Part model, mm, in its own coordinate system. Face numbers are marked on the shaded views. A direction names the side the tool comes from. Coordinates: 2 decimals unless noted, no trailing zeros. Loops run counter-clockwise (first coordinate to the right, second up) from the corner with the lowest first, then second, coordinate; pieces in that order, holes last. Notation, with made-up numbers: M 55.25,78.5 L 80.25,78.5 A16 cw 80.25,94.5 Z; hole C -24.5,-27.75 d3. An arc over 180 degrees is marked long. Use a Markdown table: item, result. Add a question column.
1) Pull direction X, two halves, no side cores. Call the marked faces 1, 2, 3 and 4: released by +X, released by -X, zero draft, split by the parting line, or undercut.
2) Tool access for the marked faces 5 and 6: list every direction of +Z, -Z, +X, -X, +Y, -Y with a clear straight run to the whole face (end or side of a thin tool).
3) Wall check: probe 1 along Z at (x, y) = (0, -54.75); probe 2 along X at (y, z) = (-6.5, -0.5); probe 3 along Z at (x, y) = (35.5, -24.5). Give the ranges that are in metal, low to high. Write a range as from..to.
4) Pin check, flat tips, straight feed: pin 1 Ø5 at (x, y) = (51.5, -20) entering from +Z; pin 2 Ø1 at (x, y) = (-0.5, -50) entering from -Z; pin 3 Ø10 at (x, y) = (35.5, -37) entering from -Z; pin 4 Ø5 at (x, z) = (0, 0) entering from -Y. Stop position of each tip, or through.
5) Band-saw the part on A-A (y = -7.5). List the corners of the cut face in (x, z).
6) Band-saw the part on B-B (x = -6). List the corners of the cut face in (y, z), plus the area to 3 significant figures.
7) Band-saw the part on D-D (z = 10.5). List the corners of the cut face in (x, y), plus the area to 3 significant figures.
8) Band-saw the part on C-C (y = -34). List the corners of the cut face in (x, z).
from build123d import *

# Parameters (mm, degrees)
F0_R           = 4
F1_DEPTH       = 58
F2_R           = 3.25
F3_DEPTH       = 13.5
F4_R           = 3.25
F5_DEPTH       = 13.5
F8_DEPTH       = 7
F8_DEPTH_BACK  = 7
F9_R           = 6.99999
F11_W          = 19
F11_H          = 3
F12_DEPTH      = 14
F17_R          = 2
F18_DEPTH      = 5
F18_DEPTH_BACK = 0.471687069
F19_R          = 2


# Not quite as in the source:
# - a fillet or chamfer is up to 0.001 mm smaller than in the source, because OpenCascade refuses the exact size


with BuildPart() as f1:
    # F0 (on Front) → F1 (new body)
    with BuildSketch(Plane.XZ):
        Circle(F0_R)
    extrude(amount=F1_DEPTH)

    # F2 (on face) → F3 (cut)
    with BuildSketch(Plane.XZ.offset(58)):
        Circle(F2_R)
    extrude(amount=-F3_DEPTH, mode=Mode.SUBTRACT)

    # F4 (on face) → F5 (cut)
    with BuildSketch(Plane(origin=(0, 0, 0), x_dir=(-1, 0, 0), z_dir=(0, 1, 0))):
        Circle(F4_R)
    extrude(amount=-F5_DEPTH, mode=Mode.SUBTRACT)

    # F7 (on offset) → F8 (join, two sides)
    with BuildSketch(Plane.XZ.offset(29)) as f8_sk:
        with BuildLine():
            Line((0, -1), (0, -4))
            Line((0, -4), (20, -4))
            ThreePointArc((20, -4), (33.4977869164, -1.9540489613), (45.7829596161, 4))
            Line((45.7829596161, 4), (89.0842298053, 29))
            Line((89.0842298053, 29), (87.5842298053, 31.5980762114))
            Line((87.5842298053, 31.5980762114), (44.1796846254, 6.5384503677))
            ThreePointArc((44.1796846254, 6.5384503677), (32.6637808585, 0.9283092986), (20, -1))
            Line((20, -1), (0, -1))
        make_face()
    extrude(amount=F8_DEPTH)
    extrude(f8_sk.sketch, amount=-F8_DEPTH_BACK)

    # F9 (radius 7 in the source; OpenCascade refuses exactly that, so slightly less here)
    f9_edges = [f1.edges().sort_by_distance(p)[0] for p in [
        (88.33423, -36, 30.299038),
        (88.33423, -22, 30.299038),
    ]]
    fillet(f9_edges, radius=F9_R)

    # F11 (on offset) → F12 (join)
    with BuildSketch(Plane(origin=(0, -5, 0), x_dir=(-1, 0, 0), z_dir=(0, 1, 0))):
        with Locations((9.5, 2.5)):
            Rectangle(F11_W, F11_H)
    extrude(amount=-F12_DEPTH)

    # F17 (on 3pt) → F18 (join, two sides)
    with BuildSketch(Plane(origin=(0.602031742, 0, -3.953721561), x_dir=(0.9886047584, 0, 0.1505344865), z_dir=(-0.1505344865, 0, 0.9886047584))) as f18_sk:
        with Locations((29.0842950344, -29.3515790254)):
            Circle(F17_R)
    extrude(amount=F18_DEPTH)
    extrude(f18_sk.sketch, amount=-F18_DEPTH_BACK)

    # F19
    f19_edges = [f1.edges().sort_by_distance(p)[0] for p in [
        (26.625022, -29.351579, 5.066423),
    ]]
    fillet(f19_edges, radius=F19_R)


solid = f1.part
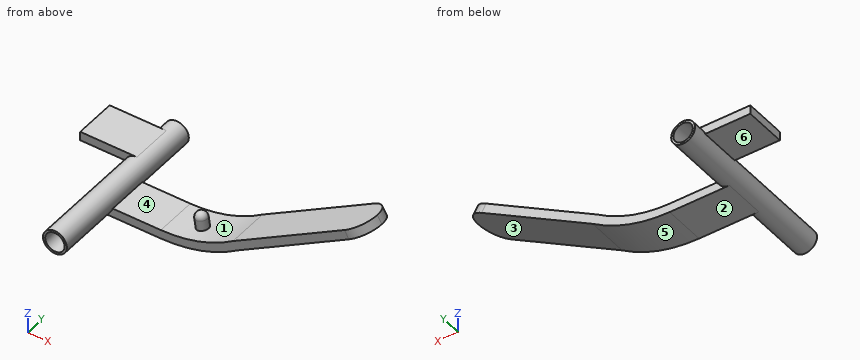
Entries:
| question | item | result |
|---|---|---|
| 1 | face 1 | undercut |
| 1 | face 2 | zero draft |
| 1 | face 3 | released by +X |
| 1 | face 4 | undercut |
| 2 | face 5 | -Z, +X, +Y, -Y |
| 2 | face 6 | -Z, -X, +Y, -Y |
| 3 | probe 1 | -4..-3.25, 3.25..4 |
| 3 | probe 2 | -3.97..-3.21, 3.21..3.97 |
| 3 | probe 3 | -1.28..1.92 |
| 4 | pin 1 | z = 11.63 |
| 4 | pin 2 | z = -4 |
| 4 | pin 3 | z = -2.75 |
| 4 | pin 4 | y = -44.5 |
| 5 | outline | M -19,1 L -3.87,1 A4 ccw long 0,4 L -19,4 Z; hole M -3.09,1 A3.25 ccw long 0,3.25 L 0,1 Z |
| 6 | outline | M -19,1 L -5,1 L -5,4 L -19,4 Z |
| 6 | area | 42.0 mm2 |
| 7 | outline | M 51.04,-36 L 57.04,-36 L 57.04,-22 L 51.04,-22 Z |
| 7 | area | 84.0 mm2 |
| 8 | outline | M 0,-4 L 20,-4 A45.55 ccw 45.78,4 L 87.26,27.95 L 85.76,30.55 L 44.18,6.54 A42.55 cw 20,-1 L 3.87,-1 A4 ccw long Z |
